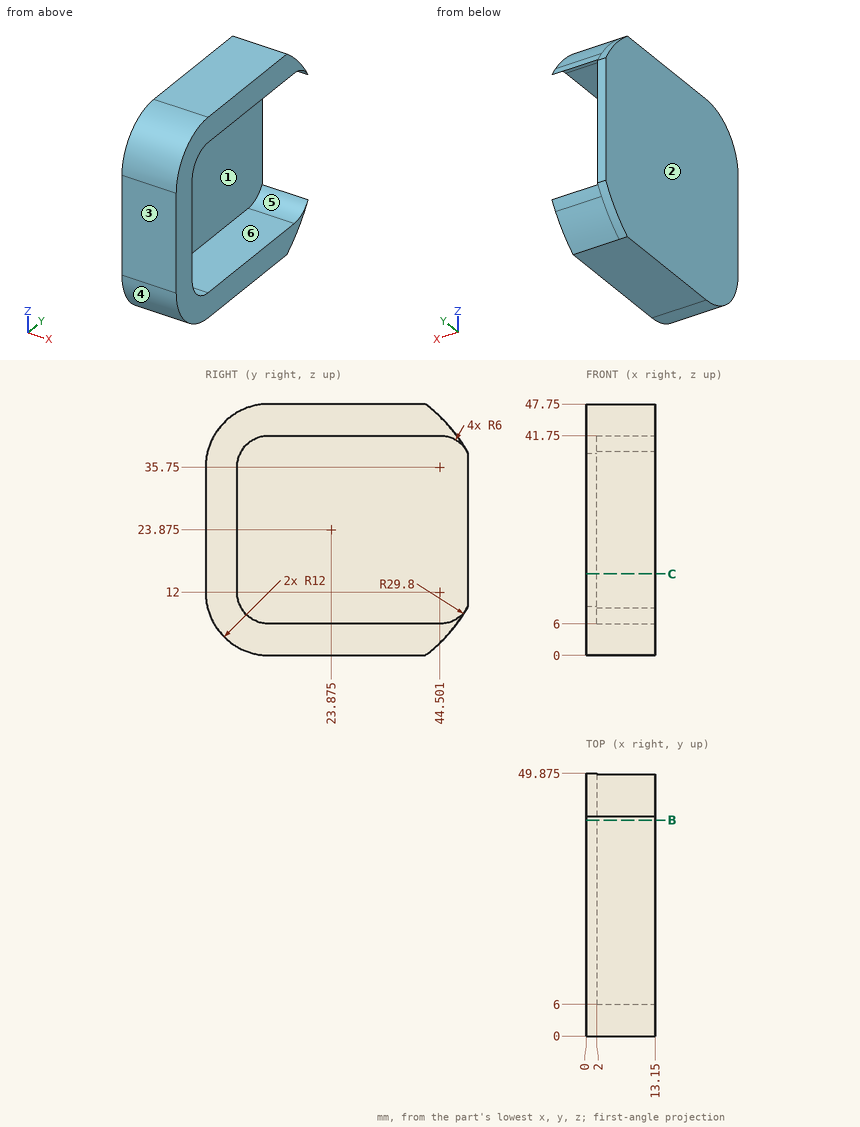
For this review, use the dimensioned drawing (mm, ordinates from the lowest corner) and the shaded views. A direction names the side the tool comes from. Round coordinates to 2 decimals unless told otherwise and drop trailing zeros. Write each loop counter-clockwise with the first axis right and the second up, starting at its lowest first coordinate (ties: lowest second). Pieces come first, ordered by that corner, then holes. Notation, with made-up numbers: M 26,49.25 L 84,49.25 A37 cw 84,85.25 Z; hole C 79.5,-12.5 d10. An arc over 180 degrees is marked long. Answer as CSV lines item,"result". Start each with the question number.
Q1. Clearance check with flat-ended pins moving along their axes: P1, Ø1, axis at y = 25.5, z = 27.5, coming from the +X side; P2, Ø3, axis at x = 11.5, y = 43.5, coming from the -Z side; P3, Ø5, axis at x = 7, z = 26.5, coming from the +Y side. State where each tip first meets the part, or that it passes through.
Q2. The part is to be moulded in two halves that separate along Z. For the marked faces 3, 4, 5 and 6, say which applies: +Z half, -Z half, draft (parallel to the pull), parting line (faces both ways), or undercut.
Q3. Consider section B-B, the plane y = 41. Give the boundary of the cut face in (x, z), then the cut area to 3 significant figures.
Q4. Consider section C-C, the plane z = 15.5. Give the boundary of the cut face in (x, y) (3 decimals), then the cut area to 3 significant figures.
Q5. Wall thickness on line 1 along Z through (x, y) = (11.5, 16); line 2 along Y through (x, z) = (2.75, 23.5); line 3 along X through (y, z) = (23, 9): over which ranges is each line inside the solid? List them lowest first.
Q6. Tool access review of the marked faces 1 and 2: name each direction out of +Z, -Z, +X, -X, +Y, -Y from which nothing blocks a thin tool from reaching the whole face with its end or side.
Result set:
1,P1,"stops at x = 2"
1,P2,"stops at z = 0.22"
1,P3,"stops at y = 6"
2,face 3,"draft"
2,face 4,"-Z half"
2,face 5,"undercut"
2,face 6,"undercut"
3,outline,"M 0,0 L 13.15,0 L 13.15,6 L 2,6 L 2,41.75 L 13.15,41.75 L 13.15,47.75 L 0,47.75 Z"
3,area,"229 mm²"
4,outline,"M 0,0 L 13.15,0 L 13.15,6 L 2,6 L 2,49.875 L 0,49.875 Z"
4,area,"167 mm²"
5,line 1,"z = 0 to 6, 41.75 to 47.75"
5,line 2,"y = 0 to 6"
5,line 3,"x = 0 to 2"
6,face 1,"+X"
6,face 2,"+Z, -Z, -X, +Y, -Y"
